Geometry check sheet. Reference: the model listing, model coordinates, mm. A direction names the side the tool comes from. Give positions to 0.01 mm unless a question says otherwise; leave off trailing zeros. Loops run counter-clockwise (first coordinate to the right, second up) from the corner with the lowest first, then second, coordinate; pieces in that order, holes last. Notation, with made-up numbers: (1.25, -15.75) -> (34.25, -15.75) arc R13 cw to (34.25, 1.25) -> close; hole circle Ø9 at (-39.5, 10). An arc over 180 degrees is marked (long way). One line per item, written item: value. Start each with the question number.
(1) Scan lines: line 1 along X through (y, z) = (4.15, 6.25); line 2 along X through (y, z) = (17, 6.25); line 3 along Z through (x, y) = (6.7, 19.9). Record each from-to range of solid material in increasing order. Write a range as from..to.
(2) Sectioned sample at D-D, the plane x = 24.5. Record the cut outline in (y, z) (3 decimals), then the cut area to 3 significant figures.
(3) Sectioned sample at B-B, the plane z = 6.25. State how many separate pieces and enclosed holes the cut face has, then the cut area to 3 significant figures.
(4) Gauge pin test, flat ends, axial feed: pin 1 Ø3 at (x, y) = (12.5, 1) entering from -Z; pin 2 Ø0.8 at (x, z) = (14, 2.5) entering from -Y; pin 3 Ø2 at (y, z) = (19.5, 3.5) entering from +X; pin 4 Ø4 at (y, z) = (12.5, 5) entering from -X. Record the tip position at first contact, or that the pin passes through.
(5) Sectioned sample at C-C, the plane y = 6.75. Record the cut outline in (x, z), then the cut area to 3 significant figures.
(6) Tool access check on faces 4 (the face through (36.8, 16, 6)), 5 (the face through (21, 1, 9.25)), 6 (the face through (9.2, 15, 6)). Record the directions out of +Z, -Z, +X, -X, +Y, -Y that give a thin tool (end or side, any length) a straight path to the whole face; none if there is none.
(7) Draft check along Y on faces 1 (the face through (34, 18.6, 6)), 2 (the face through (22.881, 4.242, 4.425)), 3 (the face through (34, 13.2, 8)). Enter one of: pulls with the +Y half, pulls with the -Y half, needs draft (parallel to the pull), parting line crosses it, or undercut.
(8) Sectioned sample at A-A, the plane x = 34.3. Record the cut outline in (y, z) (3 decimals).
Autodesk Fusion 360 part; units mm, degrees
sketch "Sketch1" plane through (0, 0, 0) normal (0, 1, 0) x (1, 0, 0)
  line L0 (0, 0) -> (41, 0)
  line L1 (41, 0) -> (41, -12.5)
  line L2 (41, -12.5) -> (0, -12.5)
  line L3 (0, -12.5) -> (0, 0)
  dimension "d1" = 41
  dimension "d2" = 12.5
extrude "Extrude1" add sketch "Sketch1" along normal blind 7.2
sketch "Sketch2" plane through (0, 0, 0) normal (0, -1, 0) x (1, 0, 0)
  line L0 (41, 12.5) -> (0, 12.5)
  line L1 (0, 12.5) -> (0, 0)
  line L2 (0, 0) -> (41, 0)
  line L3 (41, 0) -> (41, 12.5)
  line L4 (41, 9.25) -> (0, 9.25)
  line L5 (0, 9.25) -> (0, 3.25)
  line L6 (0, 3.25) -> (41, 3.25)
  line L7 (41, 3.25) -> (41, 9.25)
  dimension "d5" = 6
extrude "Extrude2" cut sketch "Sketch2" against normal blind 1.2 contours L1 L3 L4 L5 L6 L7
sketch "Sketch3" plane through (0, 7.2, 0) normal (0, 1, 0) x (-1, 0, 0)
  line L0 (0, 12.5) -> (-41, 12.5)
  line L1 (-41, 12.5) -> (-41, 0)
  line L2 (-41, 0) -> (0, 0)
  line L3 (0, 0) -> (0, 12.5)
  circle A0 centre (-20.5, 6.25) radius 3
  dimension "d8" = 6
  dimension "d9" = 6.25
  dimension "d10" = 20.5
extrude "Extrude3" cut sketch "Sketch3" against normal blind 6 contours A0
sketch "Sketch4" plane through (0, 0, 0) normal (0, -1, 0) x (1, 0, 0)
  line L0 (0, 9.25) -> (41, 9.25)
  line L1 (41, 9.25) -> (41, 12.5)
  line L2 (41, 12.5) -> (0, 12.5)
  line L3 (0, 12.5) -> (0, 9.25)
  line L4 (41, 1.625) -> (0, 1.625)
  line L5 (0, 1.625) -> (0, 10.875)
  line L6 (0, 10.875) -> (41, 10.875)
  line L7 (41, 10.875) -> (41, 1.625)
  arc A0 (20.5, 3.25) -> (20.5, 9.25) centre (20.5, 6.25) ccw
  line L8 (20.5, 3.25) -> (41, 3.25)
  line L9 (41, 3.25) -> (41, 9.25)
  line L10 (41, 9.25) -> (20.5, 9.25)
  line L11 (0, 0) -> (41, 0)
  dimension "d13" = 9.25
  dimension "d14" = 1.625
sketch "Sketch5" plane through (0, 0, 0) normal (0, -1, 0) x (1, 0, 0)
  line L0 (41, 3.25) -> (0, 3.25)
  line L1 (0, 3.25) -> (0, 0)
  line L2 (0, 0) -> (41, 0)
  line L3 (41, 0) -> (41, 3.25)
sketch "Sketch6" plane through (20.5, 0, 1.625) normal (0, -1, 0) x (1, 0, 0)
  line L0 (20.5, -1.625) -> (-20.5, -1.625)
  line L1 (-20.5, -1.625) -> (-20.5, 0)
  line L2 (-20.5, 0) -> (20.5, 0)
  line L3 (20.5, 0) -> (20.5, -1.625)
  point P0 (20.5, -1.625)
  point P1 (-20.5, 0)
extrude "Extrude4" add sketch "Sketch6" sketch "Sketch4" along normal blind 3.5 of sketch 2 contours L1 L2 L3 L6
sketch "Sketch7" plane through (0, 7.2, 0) normal (0, 1, 0) x (-1, 0, 0)
  circle A0 centre (-20.5, 6.25) radius 3
  line L0 (0, 12.5) -> (-41, 12.5)
  line L1 (-41, 12.5) -> (-41, 0)
  line L2 (-41, 0) -> (0, 0)
  line L3 (0, 0) -> (0, 12.5)
  line L4 (-4.2, 0) -> (-9.2, 0)
  line L5 (-9.2, 0) -> (-9.2, 12.5)
  line L6 (-9.2, 12.5) -> (-4.2, 12.5)
  line L7 (-4.2, 12.5) -> (-4.2, 0)
  line L8 (-36.8, 0) -> (-31.8, 0)
  line L9 (-31.8, 0) -> (-31.8, 12.5)
  line L10 (-31.8, 12.5) -> (-36.8, 12.5)
  line L11 (-36.8, 12.5) -> (-36.8, 0)
  dimension "d17" = 5
  dimension "d18" = 5
  dimension "d19" = 22.6
  dimension "d20" = 4.2
extrude "Extrude5" add sketch "Sketch7" along normal blind 15.5 contours L0 L2 L4 L5 L6 L7 | L0 L2 L8 L9 L10 L11
sketch "Sketch8" plane through (36.8, 0, 0) normal (1, 0, 0) x (0, 0, -1)
  line L0 (-12.5, 7.2) -> (0, 7.2)
  line L1 (0, 7.2) -> (0, 22.7)
  line L2 (0, 22.7) -> (-12.5, 22.7)
  line L3 (-12.5, 22.7) -> (-12.5, 7.2)
  line L4 (-12.5, 11.2) -> (-4, 11.2)
  line L5 (-4, 11.2) -> (-4, 13.2)
  line L6 (-4, 13.2) -> (-12.5, 13.2)
  line L7 (-12.5, 13.2) -> (-12.5, 11.2)
  dimension "d23" = 8.5
  dimension "d24" = 2
  dimension "d25" = 4
extrude "Extrude6" cut sketch "Sketch8" against normal blind 5 contours L3 L4 L5 L6 L7
fillet "Fillet1" radius 2.5 4 edges at (41, 7.2, 6.25) (36.8, 7.2, 6.25) (0, 7.2, 6.25) (4.2, 7.2, 6.25)
sketch "Sketch9" plane through (0, 22.7, 0) normal (0, 1, 0) x (-1, 0, 0)
  line L0 (-4.2, 12.5) -> (-9.2, 12.5)
  line L1 (-9.2, 12.5) -> (-9.2, 0)
  line L2 (-9.2, 0) -> (-4.2, 0)
  line L3 (-4.2, 0) -> (-4.2, 12.5)
  circle A0 centre (-6.7, 6.25) radius 1.75
  circle A1 centre (-34.3, 6.25) radius 1.75
  line L4 (-31.8, 0) -> (-31.8, 12.5)
  line L5 (-36.8, 0) -> (-31.8, 0)
  dimension "d30" = 3.5
  dimension "d31" = 3.5
  dimension "d32" = 2.5
  dimension "d33" = 2.5
  dimension "d34" = 6.25
  dimension "d35" = 6.25
extrude "Extrude7" cut sketch "Sketch9" against normal blind 4.1 contours A0 | A1
sketch "Sketch10" plane through (0, 0, 12.5) normal (0, 0, 1) x (1, 0, 0)
  arc A0 (2.1, 7.1678) -> (0, 4.7) centre (2.5, 4.7) ccw
  line L0 (0, 4.7) -> (0, -3.5)
  line L1 (0, -3.5) -> (41, -3.5)
  line L2 (41, -3.5) -> (41, 4.7)
  arc A1 (41, 4.7) -> (38.9, 7.1678) centre (38.5, 4.7) ccw
  arc A2 (36.8, 9.6356) -> (38.9, 7.1678) centre (39.3, 9.6356) ccw
  line L3 (36.8, 9.6356) -> (36.8, 11.2)
  line L4 (36.8, 11.2) -> (31.8, 11.2)
  line L5 (31.8, 11.2) -> (31.8, 7.2)
  line L6 (31.8, 7.2) -> (9.2, 7.2)
  line L7 (9.2, 7.2) -> (9.2, 22.7)
  line L8 (9.2, 22.7) -> (4.2, 22.7)
  line L9 (4.2, 22.7) -> (4.2, 9.6356)
  arc A3 (2.1, 7.1678) -> (4.2, 9.6356) centre (1.7, 9.6356) ccw
  line L10 (41, 1) -> (0, 1)
  line L11 (0, 1) -> (0, 3)
  line L12 (0, 3) -> (41, 3)
  line L13 (41, 3) -> (41, 1)
  dimension "d38" = 2
  dimension "d39" = 4.5
extrude "Extrude8" cut sketch "Sketch10" against normal blind 1.5 contours L0 L2 L10 L11 L12 L13
equation "d3 = 6 mm + 1.2 mm"
equation "d9 = ( 12.5 / 2 ) * 1 mm"
equation "d10 = ( 41 / 2 ) * 1 mm"
equation "d14 = ( 12.5 mm - d13 ) / 2"
equation "d20 = ( ( 41 - 32.6 ) / 2 ) * 1 mm"
equation "d25 = 5 mm - d24 / 2"
equation "d34 = ( 12.5 / 2 ) * 1 mm"
equation "d35 = d34"
equation "d39 = 2.5 mm + 2 mm"
Calculated:
1. line 1: x = 0..17.5, 23.5..41
1. line 2: x = 4.2..9.2, 31.8..36.8
1. line 3: z = 0..4.5, 8..12.5
2. outline: (-3.5, 0) -> (7.2, 0) -> (7.2, 12.5) -> (3, 12.5) -> (3, 11) -> (1, 11) -> (1, 12.5) -> (-3.5, 12.5) -> (-3.5, 10.875) -> (0, 10.875) -> (0, 9.25) -> (1.2, 9.25) -> (1.2, 3.25) -> (0, 3.25) -> (0, 1.625) -> (-3.5, 1.625) -> close
2. area: 91.2 mm2
3. separate pieces: 3
3. enclosed holes: 0
3. area: 326 mm2
4. pin 1: stops at z = 0
4. pin 2: stops at y = 0
4. pin 3: stops at x = 36.8
4. pin 4: stops at x = 4.2
5. outline: (1.07, 0) -> (39.93, 0) -> (39.93, 12.5) -> (1.07, 12.5) -> close; hole circle Ø6 at (20.5, 6.25)
5. area: 457 mm2
6. face 4: +Z, -Z, +X, +Y
6. face 5: +X, -X, -Y
6. face 6: +Z, -Z, +Y
7. face 1: pulls with the +Y half
7. face 2: needs draft
7. face 3: undercut
8. outline: (-3.5, 0) -> (22.7, 0) -> (22.7, 4.5) -> (18.6, 4.5) -> (18.6, 8) -> (22.7, 8) -> (22.7, 12.5) -> (13.2, 12.5) -> (13.2, 4) -> (11.2, 4) -> (11.2, 12.5) -> (3, 12.5) -> (3, 11) -> (1, 11) -> (1, 12.5) -> (-3.5, 12.5) -> (-3.5, 10.875) -> (0, 10.875) -> (0, 9.25) -> (1.2, 9.25) -> (1.2, 3.25) -> (0, 3.25) -> (0, 1.625) -> (-3.5, 1.625) -> close
